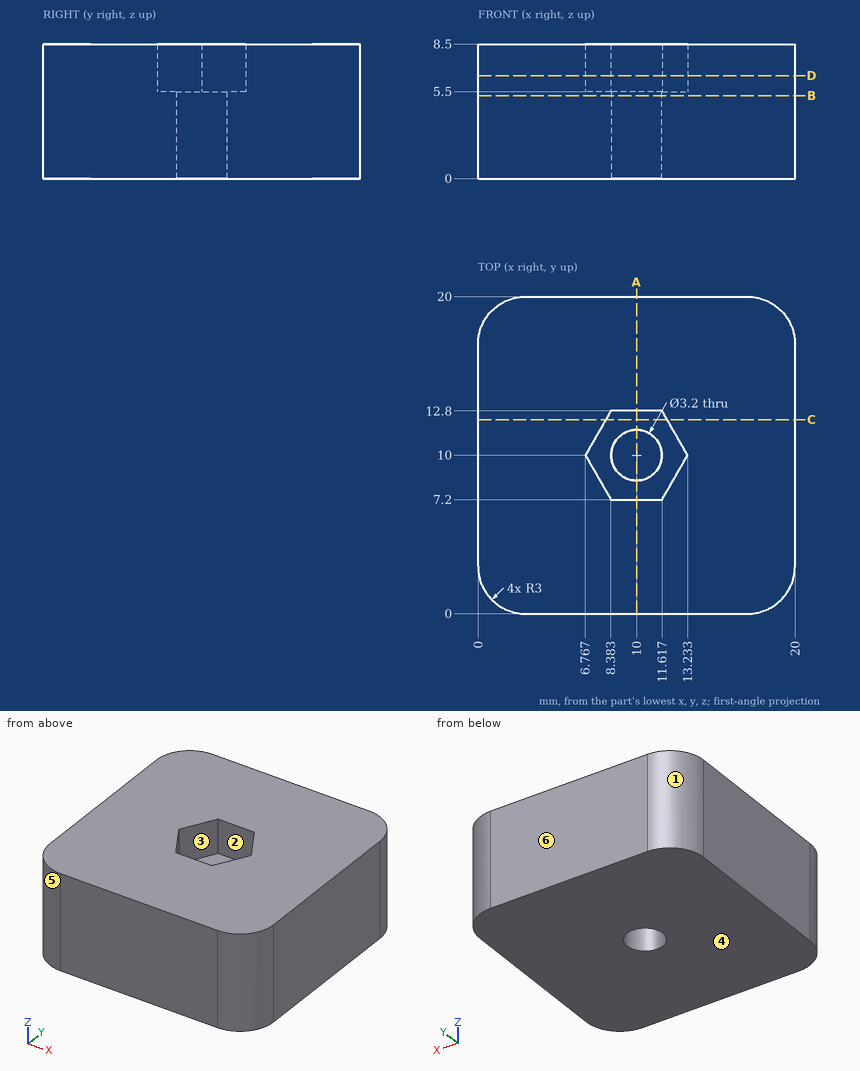
Here's the drawing with two shaded views (mm, measured from the low corner). I have some questions. A direction names the side the tool comes from. Give positions to 0.01 mm unless a question says otherwise; leave off trailing zeros. Loops run counter-clockwise (first coordinate to the right, second up) from the corner with the lowest first, then second, coordinate; pieces in that order, holes last. Notation, with made-up numbers: (-36.75, 25) - (-21.75, 25) arc R30 cw to (-21.75, 59) - close; hole circle Ø6 at (63, -12.75). An arc over 180 degrees is marked (long way). Return JSON: item names as keys, results as strings.
1. I want a section at C-C on y = 12.25. Please give me the cut outline in (x, z), and give its area (3 significant figures).
Output values:
{"outline": "(0, 0) - (20, 0) - (20, 8.5) - (11.93, 8.5) - (11.93, 5.5) - (8.07, 5.5) - (8.07, 8.5) - (0, 8.5) - close", "area": "158 mm²"}
2. If I drill on line 1 (Y direction, x = 10, z = 1.4); line 2 (Y direction, x = 8.5, z = 7.25), over which ranges is the centre line in solid material (lowest first)?
Output values:
{"line 1": "y = 0 to 8.4, 11.6 to 20", "line 2": "y = 0 to 7.2, 12.8 to 20"}
3. For the marked faces 1 and 2, which set-ups out of +Z, -Z, +X, -X, +Y, -Y let a thin tool reach every point of the face, with its end or its side?
Output values:
{"face 1": "+Z, -Z, -X, +Y", "face 2": "+Z"}
4. I want a section at D-D on z = 6.5. Please give me the cut outline in (x, y).
Output values:
{"outline": "(0, 3) arc R3 ccw to (3, 0) - (17, 0) arc R3 ccw to (20, 3) - (20, 17) arc R3 ccw to (17, 20) - (3, 20) arc R3 ccw to (0, 17) - close; hole (6.77, 10) - (8.38, 7.2) - (11.62, 7.2) - (13.23, 10) - (11.62, 12.8) - (8.38, 12.8) - close"}
5. I want a section at A-A on x = 10. Please give me the cut outline in (y, z).
Output values:
{"outline": "(0, 0) - (8.4, 0) - (8.4, 5.5) - (7.2, 5.5) - (7.2, 8.5) - (0, 8.5) - close; (11.6, 0) - (20, 0) - (20, 8.5) - (12.8, 8.5) - (12.8, 5.5) - (11.6, 5.5) - close"}
6. We'd pull the mould along Y, two halves only. Please class the marked faces 3, 4, 5 and 6: +Y half, -Y half, draft (parallel to the pull), parting line (faces both ways), or undercut.
Output values:
{"face 3": "undercut", "face 4": "draft", "face 5": "-Y half", "face 6": "+Y half"}
7. I want a section at B-B on z = 5.25. Please give me the cut outline in (x, y).
Output values:
{"outline": "(0, 3) arc R3 ccw to (3, 0) - (17, 0) arc R3 ccw to (20, 3) - (20, 17) arc R3 ccw to (17, 20) - (3, 20) arc R3 ccw to (0, 17) - close; hole circle Ø3.2 at (10, 10)"}
